Design review of the part shown in the three views and the two pictorial views. Dimensions are in mm from the part's minimum x, y and z. A direction names the side the tool comes from. Coordinates: 2 decimals unless noted, no trailing zeros. Order: outer loops, then holes, each group sorted by start corner. A loop starts at its lowest first (then second) coordinate and runs counter-clockwise, first axis right, second up. Notation, with made-up numbers: (-6, 8) - (45, 8) arc R15 cw to (45, 23) - close; hole circle Ø11 at (-7.75, 76.25). An arc over 180 degrees is marked (long way). One line per item, written item: value. Start each with the question number.
(1) Consider section A-A on y = 7.5. Write out the cut boundary in (x, z), then the cut area to 3 significant figures.
(2) Consider section D-D on z = 7.25. Write out the cut boundary in (x, y).
(3) Clearance check with flat-ended pins moving along their axes: pin 1 (1 mm diameter, centred on x = 12, z = 2.5, fed in from -Y); pin 2 (3 mm diameter, centred on x = 5.5, z = 4.5, fed in from +Y); pin 3 (4 mm diameter, centred on y = 12.5, z = 8.5, fed in from +X). State where each tip first meets the part, or that it passes through.
(4) To check wall thickness, follow line 1 along X through (y, z) = (7.25, 14.5); line 2 along Z through (x, y) = (5.25, 3) (1 decimal). State the ranges of each line that lie inside material, in increasing order.
(5) Consider section C-C on z = 1.5. Write out the cut boundary in (x, y).
(6) For the marked faces 1 and 2, list the 3-axis set-ups (+Z, -Z, +X, -X, +Y, -Y) from which the entire face can be reached by the end or side of a thin tool; tool diameter is ignored.
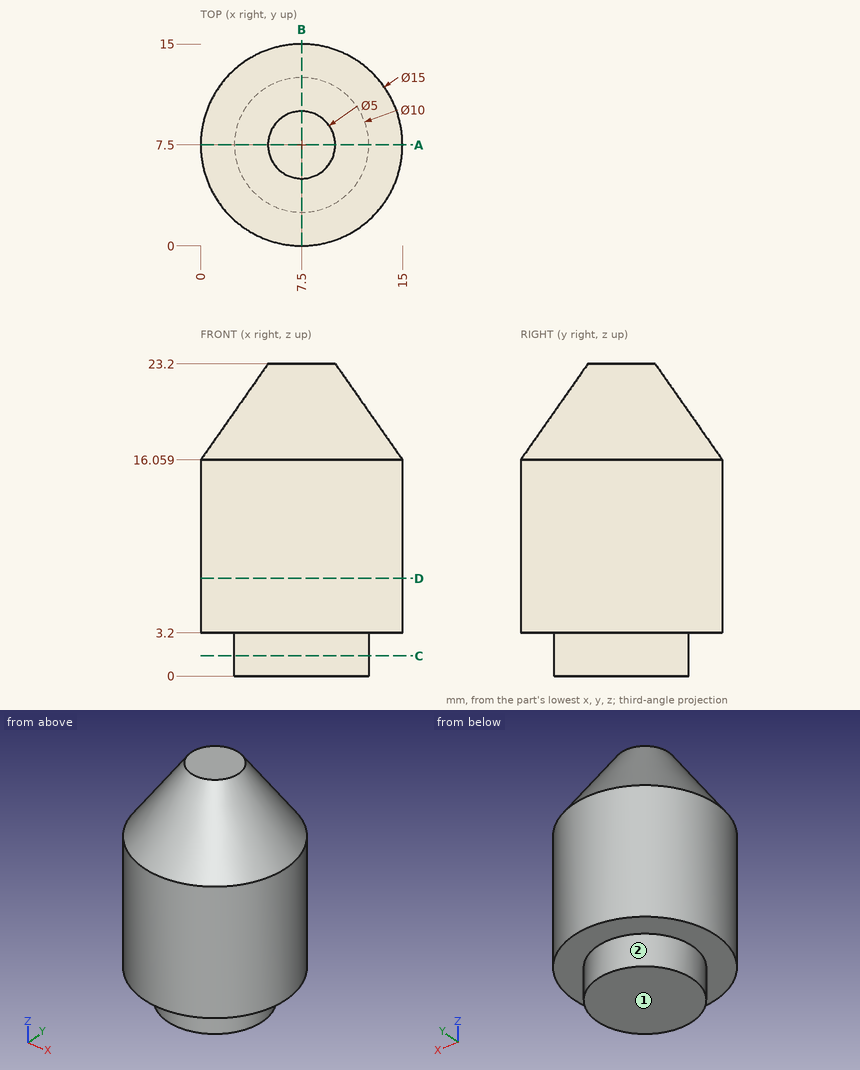
Geometry check:
1. outline: (0, 3.2) - (2.5, 3.2) - (2.5, 0) - (12.5, 0) - (12.5, 3.2) - (15, 3.2) - (15, 16.06) - (10, 23.2) - (5, 23.2) - (0, 16.06) - close
1. area: 296 mm^2
2. outline: circle Ø15 at (7.5, 7.5)
3. pin 1: stops at y = 4.5
3. pin 2: stops at y = 14.98
3. pin 3: stops at x = 14.37
4. line 1: x = 0 to 15
4. line 2: z = 3.2 to 19.6
5. outline: circle Ø10 at (7.5, 7.5)
6. face 1: -Z, +X, -X, +Y, -Y
6. face 2: -Z
